For this review, take the finished solid that the model builds, in its own axes (mm). A direction names the side the tool comes from. Give positions to 0.01 mm unless a question says otherwise; leave off trailing zeros. Write each loop counter-clockwise with the first axis right and the second up, starting at its lowest first coordinate (ties: lowest second). Pieces come first, ordered by that corner, then holes.
1) Wall thickness on line 1 along Z through (x, y) = (-6.5, 0.25); line 2 along Z through (x, y) = (-11, -6); line 3 along X through (y, z) = (-2.75, -16): over which ranges is each line inside the solid? List them lowest first.
2) Machinability: for faces 1 (the face through (0, -9.093, 6)), 2 (the face through (-7.9, -4.5, 5.5)), 3 (the face through (-0.1, 10.4, 1.182)), 4 (the face through (-3.472, -2.662, -17.823)), 5 (the face through (7.842, -4.604, 5.508)), which of the approach directions +Z, -Z, +X, -X, +Y, -Y give a long, thin tool a straight path to every point of the face, cutting with its end or side? Answer none if there is none.
3) For P1, Ø6, axis at x = -2.5, z = -13.5, coming from the -Y side (3 decimals); P2, Ø4, axis at x = 4.5, z = -17, coming from the -Y side; P3, Ø3, axis at y = 7, z = -16.5, coming from the -X side; P4, Ø4, axis at x = 0.5, y = 0.5, coming from the +Z side, all flat-tipped, find the tip position at first contact; note any pin that passes through.
4) We need section B-B on z = -31.5. Give the boundary of the cut face in (x, y) (3 decimals), and give its area (3 significant figures).
from build123d import *

# Parameters (mm, degrees)
SKETCH1_R           = 5
BOSS_EXTRUDE1_DEPTH = 40
SKETCH1_3_R         = 15
BOSS_EXTRUDE2_DEPTH = 2
BOSS_EXTRUDE3_DEPTH = 10
CUT_EXTRUDE1_START  = 10
SKETCH2_3_R         = 5
CUT_EXTRUDE1_DEPTH  = 2
FILLET1_R           = 0.5
FILLET2_R           = 1
FILLET3_R           = 2
FILLET4_R           = 2
SCALE1_SCALE        = 0.875


with BuildPart() as part:
    # Sketch1 → Boss-Extrude1 (new body)
    with BuildSketch(Plane(origin=(0, 0, 0), x_dir=(0, 1, 0), z_dir=(0, 0, 1))):
        with Locations(Location((0, 0, 0), (0, 0, 270))):
            Circle(SKETCH1_R)
    extrude(amount=-BOSS_EXTRUDE1_DEPTH)

    # Sketch1<3> → Boss-Extrude2 (add)
    with BuildSketch(Plane(origin=(0, 0, 0), x_dir=(0, 1, 0), z_dir=(0, 0, 1))):
        with Locations(Location((0, 0, 0), (0, 0, 270))):
            Circle(SKETCH1_3_R)
    extrude(amount=BOSS_EXTRUDE2_DEPTH)

    # Sketch2 → Boss-Extrude3 (add)
    with BuildSketch(Plane.XY.offset(2)):
        Polygon((-12, 0), (-6, -10.392304845), (6, -10.392304845), (12, 0), (6, 10.392304845), (-6, 10.392304845), align=None)
    extrude(amount=BOSS_EXTRUDE3_DEPTH)

    # Sketch2<3> → Cut-Extrude1 (cut)
    with BuildSketch(Plane.XY.offset(2).offset(CUT_EXTRUDE1_START)):
        Circle(SKETCH2_3_R)
    extrude(amount=-CUT_EXTRUDE1_DEPTH, mode=Mode.SUBTRACT)

    # Fillet1
    fillet1_edges = [part.edges().sort_by_distance(p)[0] for p in [
        (-15, 0, 0),
        (-15, 0, 2),
    ]]
    fillet(fillet1_edges, radius=FILLET1_R)

    # Fillet2
    fillet2_edges = [part.edges().sort_by_distance(p)[0] for p in [
        (0, -10.392304845, 2),
        (-6, -10.392304845, 7),
        (9, -5.196152423, 2),
        (6, -10.392304845, 7),
        (9, 5.196152423, 2),
        (12, 0, 7),
        (0, 10.392304845, 2),
        (6, 10.392304845, 7),
        (-9, 5.196152423, 2),
        (-6, 10.392304845, 7),
        (-9, -5.196152423, 2),
        (-12, 0, 7),
        (0, -10.392304845, 12),
        (9, -5.196152423, 12),
        (9, 5.196152423, 12),
        (0, 10.392304845, 12),
        (-9, 5.196152423, 12),
        (-9, -5.196152423, 12),
    ]]
    fillet(fillet2_edges, radius=FILLET2_R)

    # Fillet3
    fillet3_edges = [part.edges().sort_by_distance(p)[0] for p in [
        (-5, 0, 10),
    ]]
    fillet(fillet3_edges, radius=FILLET3_R - 0.0001)  # a hair under: the kernel refuses the full size

    # Fillet4
    fillet4_edges = [part.edges().sort_by_distance(p)[0] for p in [
        (-5, 0, 12),
    ]]
    fillet(fillet4_edges, radius=FILLET4_R)


with BuildPart() as part_1:
    # Scale1: scaled about (-9e-09, 0, -4.545352594)
    add(part.part.scale(SCALE1_SCALE).moved(Location((-1e-09, 0, -0.568169074))))


solid = part_1.part
Results list:
1. line 1: z = -0.57 to 9.93
1. line 2: z = -0.57 to 1.18
1. line 3: x = -3.4 to 3.4
2. face 1: +Z, +X, -X, -Y
2. face 2: +Z, -X, -Y
2. face 3: +Z
2. face 4: -Z
2. face 5: +Z, +X, -Y
3. P1: stops at y = -4.375
3. P2: stops at y = -3.59
3. P3: passes through
3. P4: stops at z = 8.18
4. outline: circle Ø8.75 at (0, 0)
4. area: 60.1 mm2
